Input: dimensioned drawing with shaded views. Units: mm. Origin: part minimum x, y, z. Give positions to 0.01 mm unless a question says otherwise; leave off trailing zeros. Order: outer loops, then holes, each group sorted by start corner. A loop starts at its lowest first (then second) coordinate and runs counter-clockwise, first axis right, second up.
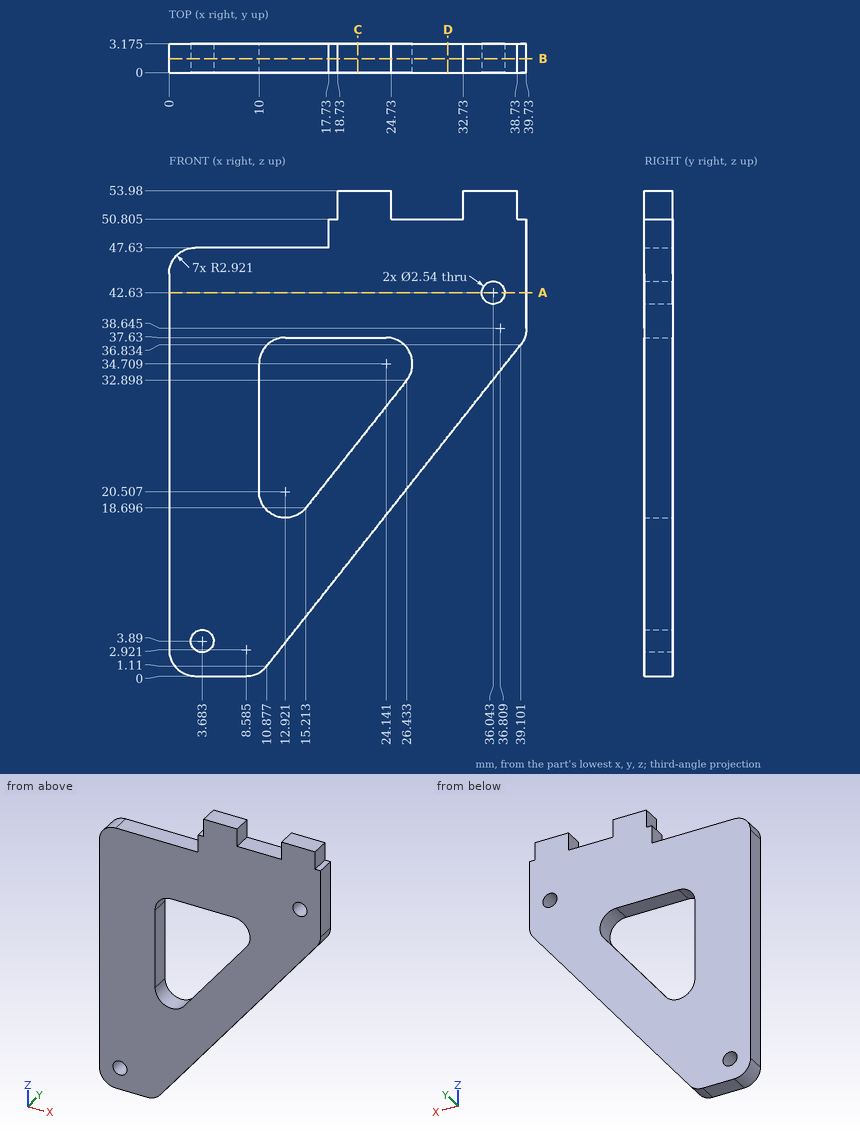
1) Material intervals for L1, parallel to Z at x = 36, y = 2.5; L2, parallel to X at y = 1.05, z = 42.63; L3, parallel to X at y = 1.75, z = 3 (1 decimal), sorted ascending.
Report:
L1: z = 32.91 to 41.36, 43.9 to 53.98
L2: x = 0 to 34.77, 37.31 to 39.73
L3: x = 0 to 2.8, 4.6 to 12.4
2) Section query C-C, the plane x = 21. Return the cut outline in (y, z) (1 decimal).
Report:
outline: (0, 13.9) - (3.2, 13.9) - (3.2, 26) - (0, 26) - close; (0, 37.6) - (3.2, 37.6) - (3.2, 54) - (0, 54) - close
3) Section query A-A, the plane z = 42.63. Return the cut outline in (x, y) (1 decimal), and give its area (3 significant figures).
Report:
outline: (0, 0) - (34.8, 0) - (34.8, 3.2) - (0, 3.2) - close; (37.3, 0) - (39.7, 0) - (39.7, 3.2) - (37.3, 3.2) - close
area: 118 mm2
4) Pin query (flat end, axial travel): pin 1 (1.6 mm diameter, centred on y = 1, z = 49, fed in from -X); pin 2 (1 mm diameter, centred on y = 2, z = 52.5, fed in from +X); pin 3 (1.6 mm diameter, centred on y = 1.5, z = 27, fed in from +X) (1 decimal). Return the tip coordinate at first contact, or that it passes through.
Report:
pin 1: stops at x = 17.73
pin 2: stops at x = 38.73
pin 3: stops at x = 32
5) Section query B-B, the plane y = 1.55. Return the cut outline in (x, z) (1 decimal), and give its area (3 significant figures).
Report:
outline: (0, 2.9) arc R2.9 ccw to (2.9, 0) - (8.6, 0) arc R2.9 ccw to (10.9, 1.1) - (39.1, 36.8) arc R2.9 ccw to (39.7, 38.6) - (39.7, 50.8) - (38.7, 50.8) - (38.7, 54) - (32.7, 54) - (32.7, 50.8) - (24.7, 50.8) - (24.7, 54) - (18.7, 54) - (18.7, 50.8) - (17.7, 50.8) - (17.7, 47.6) - (2.9, 47.6) arc R2.9 ccw to (0, 44.7) - close; hole circle Ø2.5 at (3.7, 3.9); hole (10, 20.5) arc R2.9 ccw to (15.2, 18.7) - (26.4, 32.9) arc R2.9 ccw to (24.1, 37.6) - (12.9, 37.6) arc R2.9 ccw to (10, 34.7) - close; hole circle Ø2.5 at (36, 42.6)
area: 1,190 mm2
6) Section query D-D, the plane x = 31. Return the cut outline in (y, z) (1 decimal).
Report:
outline: (0, 26.6) - (3.2, 26.6) - (3.2, 50.8) - (0, 50.8) - close
